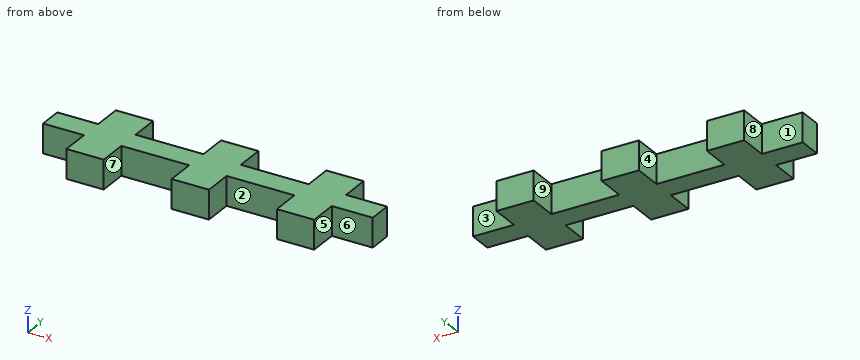
from build123d import *

# Parameters (mm, degrees)
SKETCH1_W           = 4
SKETCH1_H           = 3.175
SKETCH1_W_2         = 42.3
SKETCH1_H_2         = 2.5
BOSS_EXTRUDE1_DEPTH = 3.175
CUT_EXTRUDE2_DEPTH  = 23.175
BOSS_EXTRUDE2_DEPTH = 3.175


with BuildPart() as part:
    # Sketch1 → Boss-Extrude1 (new body)
    with BuildSketch(Plane.XY):
        with Locations((-11.5, -1.5875)):
            Rectangle(SKETCH1_W, SKETCH1_H)
        with Locations((-11.5, 4.0875)):
            Rectangle(SKETCH1_W, SKETCH1_H)
        with Locations((0, 4.0875)):
            Rectangle(SKETCH1_W, SKETCH1_H)
        with Locations((0, -1.5875)):
            Rectangle(SKETCH1_W, SKETCH1_H)
        with Locations((11.5, 4.0875)):
            Rectangle(SKETCH1_W, SKETCH1_H)
        with Locations((11.5, -1.5875)):
            Rectangle(SKETCH1_W, SKETCH1_H)
        with Locations((0, 1.25)):
            Rectangle(SKETCH1_W_2, SKETCH1_H_2)
    extrude(amount=BOSS_EXTRUDE1_DEPTH)

    # Sketch2 → Cut-Extrude2 (cut)
    with BuildSketch(Plane(origin=(0, 2.5, 0), x_dir=(1, 0, 0), z_dir=(0, 1, 0))):
        Polygon((-17.975, 0), (-21.15, 0), (-21.15, -3.175), align=None)
        Polygon((-17.975, -3.175), (-17.975, 0), (-21.15, -3.175), align=None)
        Polygon((21.15, -3.175), (17.975, -3.175), (17.975, 0), align=None)
        Polygon((21.15, -3.175), (17.975, 0), (21.15, 0), align=None)
    extrude(amount=-CUT_EXTRUDE2_DEPTH, mode=Mode.SUBTRACT)

    # Sketch3 → Boss-Extrude2 (add)
    with BuildSketch(Plane.XY.offset(3.175)):
        Polygon((-13.54064, 2.54064), (-18.01564, 2.54064), (-18.01564, -0.04064), (-13.54064, -0.04064), (-13.54064, -3.21564), (-9.45936, -3.21564), (-9.45936, -0.04064), (-2.04064, -0.04064), (-2.04064, -3.21564), (2.04064, -3.21564), (2.04064, -0.04064), (9.45936, -0.04064), (9.45936, -3.21564), (13.54064, -3.21564), (13.54064, -0.04064), (18.01564, -0.04064), (18.01564, 2.54064), (13.54064, 2.54064), (13.54064, 5.71564), (9.45936, 5.71564), (9.45936, 2.54064), (2.04064, 2.54064), (2.04064, 5.71564), (-2.04064, 5.71564), (-2.04064, 2.54064), (-9.45936, 2.54064), (-9.45936, 5.71564), (-13.54064, 5.71564), align=None)
    extrude(amount=-BOSS_EXTRUDE2_DEPTH)


solid = part.part
The listing builds one solid part. Answer for the finished solid, in the listing's coordinates (mm). Face numbers are marked on the shaded views. A direction names the side the tool comes from. Round coordinates to 2 decimals unless told otherwise and drop trailing zeros. Loops run counter-clockwise (first coordinate to the right, second up) from the corner with the lowest first, then second, coordinate; pieces in that order, holes last. Notation, with made-up numbers: M 25.5,-31 L 74.5,-31 A23 cw 74.5,-14 Z; hole C 23.25,-33 d4. An arc over 180 degrees is marked long. Return JSON: item names as keys, results as strings.
Q1. Find section C-C, the plane x = -7.5. Determine the outline of the cut face in (y, z) (3 decimals).
Results list:
{"outline": "M -0.041,0 L 2.541,0 L 2.541,3.175 L -0.041,3.175 Z"}
Q2. Find section B-B, the plane z = 2.55. Determine the outline of the cut face in (x, y).
Results list:
{"outline": "M -18.02,-0.04 L -13.54,-0.04 L -13.54,-3.22 L -9.46,-3.22 L -9.46,-0.04 L -2.04,-0.04 L -2.04,-3.22 L 2.04,-3.22 L 2.04,-0.04 L 9.46,-0.04 L 9.46,-3.22 L 13.54,-3.22 L 13.54,-0.04 L 18.02,-0.04 L 18.02,2.54 L 13.54,2.54 L 13.54,5.72 L 9.46,5.72 L 9.46,2.54 L 2.04,2.54 L 2.04,5.72 L -2.04,5.72 L -2.04,2.54 L -9.46,2.54 L -9.46,5.72 L -13.54,5.72 L -13.54,2.54 L -18.02,2.54 Z"}
Q3. Each of these flat-tipped pins is pushed along its axis until it touches: pin 1 Ø1.6 at (y, z) = (-1.5, 1) entering from +X; pin 2 Ø1.5 at (x, z) = (-3, 1.5) entering from +Y; pin 3 Ø1 at (x, z) = (5, 2.5) entering from -Y. Where does it stop, or does it pass through?
Results list:
{"pin 1": "stops at x = 13.54", "pin 2": "stops at y = 2.54", "pin 3": "stops at y = -0.04"}
Q4. Find the intervals of material crossed by line 1 along X through (y, z) = (-1.5, 1.1); line 2 along Y through (x, z) = (-6.5, 2.2), in increasing order. Write a range as from..to.
Results list:
{"line 1": "x = -13.54..-9.46, -2.04..2.04, 9.46..13.54", "line 2": "y = -0.04..2.54"}
Q5. The mould has two halves that part along X. Classify the marked faces 6, 7, 8 and 9: released by +X, released by -X, zero draft, split by the parting line, or undercut.
Results list:
{"face 6": "zero draft", "face 7": "undercut", "face 8": "released by -X", "face 9": "undercut"}
Q6. Find section A-A, the plane y = 3.5. Determine the outline of the cut face in (x, z) (3 decimals), plus the area to 3 significant figures.
Results list:
{"outline": "M -13.541,0 L -9.459,0 L -9.459,3.175 L -13.541,3.175 Z; M -2.041,0 L 2.041,0 L 2.041,3.175 L -2.041,3.175 Z; M 9.459,0 L 13.541,0 L 13.541,3.175 L 9.459,3.175 Z", "area": "38.9 mm2"}
Q7. Which of the six approach directions +Z, -Z, +X, -X, +Y, -Y give full straight-line access (tool end or side, diameter ignored) to the marked faces 1, 2, 3, 4 and 5?
Results list:
{"face 1": "+Z, -Z, -X, +Y", "face 2": "+Z, -Z, -Y", "face 3": "+Z, -Z, +X, +Y", "face 4": "+Z, -Z, +Y", "face 5": "+Z, -Z, +X, -Y"}
